Design review of the part built by this model. Coordinates are the model's own, in mm. A direction names the side the tool comes from. Give positions to 0.01 mm unless a question says otherwise; leave off trailing zeros. Loops run counter-clockwise (first coordinate to the right, second up) from the corner with the lowest first, then second, coordinate; pieces in that order, holes last. Notation, with made-up numbers: (70.25, 72.5) -> (94.25, 72.5) arc R23 ccw to (94.25, 110.5) -> close; hole circle Ø5 at (-28, 28.5). An arc over 180 degrees is marked (long way). Answer in a Markdown table with one row per item. Add a question column.
(1) Consider section A-A on y = -1.5. Write out the cut boundary in (x, z).
(2) Draft analysis for pull direction Z (two halves, no side actions). For faces 1 (the cylindrical face through (9.965, 16.86, 1.185)), 2 (the cylindrical face through (-0.04, 15.09, 1.08)), 3 (the cylindrical face through (9.96, 15.09, 1.08)), 4 (the flat face through (-5, 14.1, 1)), state which applies: +Z half, -Z half, draft (parallel to the pull), parting line (faces both ways), or undercut.
(3) For faces 5 (the flat face through (2.5, 15, 0.9)), 6 (the flat face through (0, 0, 2)), 7 (the flat face through (9.899, 14.86, 0.254)), list the 3-axis set-ups (+Z, -Z, +X, -X, +Y, -Y) from which the entire face can be reached by the end or side of a thin tool; tool diameter is ignored.
(4) Consider section C-C on x = -10.5. Write out the cut boundary in (y, z).
(5) Consider section B-B on x = 4.25. Write out the cut boundary in (y, z), then the cut area to 3 significant figures.
(6) For line 1 (Z direction, x = 7.25, y = -5.5); line 2 (Y direction, x = 1.25, z = 1.8); line 3 (Y direction, x = 4, z = 0.9), list the stretches that pass through material, from the lowest coordinate up.
(7) For pin 1 (2 mm diameter, centred on x = 0.5, y = -7.5, fed in from -Z); pin 2 (7.5 mm diameter, centred on x = -1.5, y = 1.5, fed in from +Z); pin 3 (2 mm diameter, centred on x = 6, z = 0.5, fed in from +Y); pin 4 (1.5 mm diameter, centred on x = 8, z = 3, fed in from -Y), all flat-tipped, find the tip position at first contact; note any pin that passes through.
from build123d import *

# Parameters (mm, degrees)
SKETCH1_W           = 25
SKETCH1_H           = 28.2
BOSS_EXTRUDE1_DEPTH = 2
BOSS_EXTRUDE2_DEPTH = 5
LPATTERN1_COUNT     = 3
LPATTERN1_PITCH     = 10
SKETCH6_R           = 1.050000034
CUT_EXTRUDE1_DEPTH  = 31.490326335
FILLET1_R           = 1
FILLET2_R           = 1
SKETCH7_W           = 1.937328833
SKETCH7_H           = 1.211322367
CUT_EXTRUDE2_DEPTH  = 31.490326484
FILLET7_R           = 0.254


with BuildPart() as part:
    # Sketch1 → Boss-Extrude1 (new body)
    with BuildSketch(Plane.XY):
        Rectangle(SKETCH1_W, SKETCH1_H)
    extrude(amount=BOSS_EXTRUDE1_DEPTH)

    # Sketch5 → Boss-Extrude2 (add)
    with BuildSketch(Plane.ZY.offset(12.5)):
        with BuildLine():
            Line((0.5, 15.6), (0, 14.1))
            Line((0, 14.1), (2, 14.1))
            ThreePointArc((2, 14.1), (3.060660172, 16.660660172), (0.5, 15.6))
        make_face()
    boss_extrude2 = extrude(amount=-BOSS_EXTRUDE2_DEPTH)

    # LPattern1: Boss-Extrude2 ×3
    with Locations(*[(i * LPATTERN1_PITCH, 0, 0) for i in range(1, LPATTERN1_COUNT)]):
        add(boss_extrude2)

    # Sketch6 → Cut-Extrude1 (cut, through all)
    with BuildSketch(Plane.ZY.offset(12.5)):
        with Locations((2, 15.6)):
            Circle(SKETCH6_R)
    extrude(amount=-CUT_EXTRUDE1_DEPTH, mode=Mode.SUBTRACT)

    # Fillet1
    # the kernel refuses this fillet: 1 mm, written as the material it takes off along each edge
    with BuildSketch(Plane(origin=(12.5, -20.1, 0), x_dir=(0, 0, 1), z_dir=(0, 1, 0)), Plane(origin=(-12.5, 20.1, 0), x_dir=(0, 0, 1), z_dir=(0, -1, 0))) as fillet1_piece_1:
        with BuildLine():
            CenterArc((FILLET1_R, -FILLET1_R), FILLET1_R, 90, 90)
            Line((0, -FILLET1_R), (-FILLET1_R * 0.02, -FILLET1_R))
            Line((-FILLET1_R * 0.02, -FILLET1_R), (-FILLET1_R * 0.02, FILLET1_R * 0.02))
            Line((-FILLET1_R * 0.02, FILLET1_R * 0.02), (FILLET1_R, FILLET1_R * 0.02))
            Line((FILLET1_R, FILLET1_R * 0.02), (FILLET1_R, 0))
        make_face()
    extrude(amount=40.2, mode=Mode.SUBTRACT)
    with BuildSketch(Plane(origin=(-18.5, -14.1, 0), x_dir=(0, 0, 1), z_dir=(1, 0, 0))) as fillet1_piece_2:
        with BuildLine():
            CenterArc((FILLET1_R, -FILLET1_R), FILLET1_R, 90, 90)
            Line((0, -FILLET1_R), (-FILLET1_R * 0.02, -FILLET1_R))
            Line((-FILLET1_R * 0.02, -FILLET1_R), (-FILLET1_R * 0.02, FILLET1_R * 0.02))
            Line((-FILLET1_R * 0.02, FILLET1_R * 0.02), (FILLET1_R, FILLET1_R * 0.02))
            Line((FILLET1_R, FILLET1_R * 0.02), (FILLET1_R, 0))
        make_face()
    extrude(amount=37, mode=Mode.SUBTRACT)

    # Fillet2
    # the kernel refuses this fillet: 1 mm, written as the material it takes off along each edge
    with BuildSketch(Plane(origin=(-11.5, -13.1, 1), x_dir=(-1, 0, 0), z_dir=(0, -1, 0))) as fillet2_piece_1_section:
        Polygon((0, 0), (FILLET2_R, 0), (FILLET2_R, FILLET2_R), (0, FILLET2_R), align=None)
    fillet2_piece_1 = extrude(amount=FILLET2_R, mode=Mode.PRIVATE)
    fillet2_piece_1 = fillet2_piece_1 - Plane(origin=(-11.5, -13.1, 1), x_dir=(0.7071067811865475, 0, 0.7071067811865475), z_dir=(0, -1, 0)) * Sphere(FILLET2_R, mode=Mode.PRIVATE)
    add(fillet2_piece_1, mode=Mode.SUBTRACT)
    with BuildSketch(Plane(origin=(11.5, -13.1, 1), x_dir=(1, 0, 0), z_dir=(0, -1, 0))) as fillet2_piece_2_section:
        Polygon((0, 0), (FILLET2_R, 0), (FILLET2_R, -FILLET2_R), (0, -FILLET2_R), align=None)
    fillet2_piece_2 = extrude(amount=FILLET2_R, mode=Mode.PRIVATE)
    fillet2_piece_2 = fillet2_piece_2 - Plane(origin=(11.5, -13.1, 1), x_dir=(-0.7071067811865475, 0, 0.7071067811865475), z_dir=(0, -1, 0)) * Sphere(FILLET2_R, mode=Mode.PRIVATE)
    add(fillet2_piece_2, mode=Mode.SUBTRACT)
    with BuildSketch(Plane(origin=(12.5, -14.1, 1), x_dir=(-1, 0, 0), z_dir=(0, 0, 1))) as fillet2_piece_3:
        with BuildLine():
            CenterArc((FILLET2_R, -FILLET2_R), FILLET2_R, 90, 90)
            Line((0, -FILLET2_R), (0, 0))
            Line((0, 0), (FILLET2_R, 0))
        make_face()
    extrude(amount=3.5, mode=Mode.SUBTRACT)
    with BuildSketch(Plane(origin=(-12.5, -14.1, 1), x_dir=(1, 0, 0), z_dir=(0, 0, 1))) as fillet2_piece_4:
        with BuildLine():
            CenterArc((FILLET2_R, FILLET2_R), FILLET2_R, 180, 90)
            Line((0, FILLET2_R), (0, 0))
            Line((0, 0), (FILLET2_R, 0))
        make_face()
    extrude(amount=3.5, mode=Mode.SUBTRACT)

    # Sketch7 → Cut-Extrude2 (cut, through all)
    with BuildSketch(Plane.ZY.offset(12.5)):
        with Locations((3.702300239, 16.302688342)):
            Rectangle(SKETCH7_W, SKETCH7_H)
    extrude(amount=-CUT_EXTRUDE2_DEPTH, mode=Mode.SUBTRACT)

    # Fillet7
    # the kernel refuses this fillet: 0.254 mm, written as the material it takes off along each edge
    with BuildSketch(Plane(origin=(-6.784662672, 15.697027158, 3.496858621), x_dir=(0, -0.999525916105083, -0.03078868354273752), z_dir=(-1, 0, 0))) as fillet7_piece_1:
        with BuildLine():
            CenterArc((0.26190884, -0.252842039), FILLET7_R, 84.526905726, 97.237434721)
            Line((0.008029258, -0.260662364), (0, 0))
            ThreePointArc((0, 0), (0.143067466, 0.006838354), (0.286134931, 0))
        make_face()
    extrude(amount=6.430674656, mode=Mode.SUBTRACT)
    with BuildSketch(Plane(origin=(-6.877474788, 15.697027158, 3.045507437), x_dir=(0, 0, 1), z_dir=(-1, 0, 0))) as fillet7_piece_2:
        with BuildLine():
            CenterArc((0.249010085, -0.254), FILLET7_R, 90, 83.086084758)
            ThreePointArc((-0.003142862, -0.223424002), (0.004388728, -0.111795842), (0, 0))
            Line((0, 0), (0.249010085, 0))
        make_face()
    extrude(amount=6.245050424, mode=Mode.SUBTRACT)
    with BuildSketch(Plane(origin=(-6.34649613, 16.351184765, 2.733635822), x_dir=(0, 1, 0), z_dir=(-1, 0, 0)), Plane(origin=(13.65350387, 16.351184765, 2.733635822), x_dir=(0, 1, 0), z_dir=(-1, 0, 0)), Plane(origin=(3.65350387, 16.351184765, 2.733635822), x_dir=(0, 1, 0), z_dir=(-1, 0, 0))) as fillet7_piece_3:
        with BuildLine():
            CenterArc((0.461401548, 0.254), FILLET7_R, 158.418835743, 111.581164257)
            ThreePointArc((0.225207594, 0.347425994), (0.129898026, 0.162502575), (0, 0))
            Line((0, 0), (0.461401548, 0))
        make_face()
    extrude(amount=7.30700774, mode=Mode.SUBTRACT)
    with BuildSketch(Plane(origin=(-12.934394729, 16.908349525, 2.733635822), x_dir=(0, -1, 0), z_dir=(1, 0, 0)), Plane(origin=(7.065605271, 16.908349525, 2.733635822), x_dir=(0, -1, 0), z_dir=(1, 0, 0)), Plane(origin=(-2.934394729, 16.908349525, 2.733635822), x_dir=(0, -1, 0), z_dir=(1, 0, 0))) as fillet7_piece_4:
        with BuildLine():
            CenterArc((0.158364535, 0.254), FILLET7_R, 202.640044459, 67.359955541)
            ThreePointArc((-0.076062582, 0.156225121), (-0.040295304, 0.077010263), (0, 0))
            Line((0, 0), (0.158364535, 0))
        make_face()
    extrude(amount=5.868789458, mode=Mode.SUBTRACT)
    with BuildSketch(Plane(origin=(13.215337328, 15.697027158, 3.496858621), x_dir=(0, 0, -1), z_dir=(-1, 0, 0)), Plane(origin=(3.215337328, 15.697027158, 3.496858621), x_dir=(0, 0, -1), z_dir=(-1, 0, 0))) as fillet7_piece_5:
        with BuildLine():
            CenterArc((0.260785999, 0.254), FILLET7_R, 172.762565279, 97.237434721)
            ThreePointArc((0.008809718, 0.285999279), (-0.002430253, 0.143210184), (0, 0))
            Line((0, 0), (0.260785999, 0))
        make_face()
    extrude(amount=6.430674656, mode=Mode.SUBTRACT)
    with BuildSketch(Plane(origin=(13.122525212, 15.697027158, 3.045507437), x_dir=(0, -0.999901077195103, -0.014065412332113414), z_dir=(-1, 0, 0)), Plane(origin=(3.122525212, 15.697027158, 3.045507437), x_dir=(0, -0.999901077195103, -0.014065412332113414), z_dir=(-1, 0, 0))) as fillet7_piece_6:
        with BuildLine():
            CenterArc((0.250472444, 0.252558067), FILLET7_R, 180.805915338, 83.086084758)
            Line((-0.00350243, 0.248985452), (0, 0))
            ThreePointArc((0, 0), (0.111723053, 0.005960748), (0.223446106, 0))
        make_face()
    extrude(amount=6.245050424, mode=Mode.SUBTRACT)


solid = part.part
Values follow:
| question | item | result |
|---|---|---|
| 1 | outline | (-12.5, 1) arc R1 ccw to (-11.5, 0) -> (11.5, 0) arc R1 ccw to (12.5, 1) -> (12.5, 2) -> (-12.5, 2) -> close |
| 2 | face 1 | parting line |
| 2 | face 2 | undercut |
| 2 | face 3 | undercut |
| 2 | face 4 | draft |
| 3 | face 5 | +Z, -Z, +Y |
| 3 | face 6 | +Z, +X, -X, -Y |
| 3 | face 7 | -Z, +X, -X, +Y |
| 4 | outline | (-14.1, 1) arc R1 ccw to (-13.1, 0) -> (14.1, 0) -> (15.6, 0.5) arc R1.5 ccw to (16.98, 2.58) arc R0.25 ccw to (16.78, 2.73) arc R0.25 ccw to (16.58, 2.39) arc R1.05 cw (long way) to (15.47, 3.04) arc R0.25 ccw to (15.7, 3.27) arc R0.25 ccw to (15.41, 3.49) arc R1.5 ccw to (14.1, 2) -> (-14.1, 2) -> close |
| 5 | outline | (-14.1, 1) arc R1 ccw to (-13.1, 0) -> (14.1, 0) -> (14.1, 2) -> (-14.1, 2) -> close |
| 5 | area | 56.2 mm2 |
| 6 | line 1 | 0 to 2 |
| 6 | line 2 | -14.1 to 14.57, 16.63 to 17.09 |
| 6 | line 3 | -14.09 to 14.1 |
| 7 | pin 1 | z = 0 |
| 7 | pin 2 | z = 2 |
| 7 | pin 3 | y = 14.1 |
| 7 | pin 4 | y = 14.12 |
